Autodesk Inventor part; units mm, degrees
ref_plane "Work Plane1" through (0, 0, 1.6) normal (0, 0, 1) x (1, 0, 0)
ref_plane "Work Plane2" through (15, 0, 0) normal (1, 0, 0) x (0, 1, 0)
ref_plane "XZ Plane" through (0, 0, 0) normal (0, 1, 0) x (-1, 0, 0)
sketch "Sketch2" plane through (0, 0, 0) normal (0, 1, 0) x (-1, 0, 0)
  line L0 (0, 0) -> (-5, 0)
  line L1 (-5, 0) -> (-10, 1.6)
  line L2 (-10, 1.6) -> (-15, 1.6)
  dimension "d0" = 1.6
  dimension "d1" = 5
  dimension "d2" = 5
  dimension "d3" = 5
sketch "Sketch3" plane through (0, 0, 0) normal (1, 0, 0) x (0, 1, 0)
  circle A0 centre (0, 0) radius 0.9
  dimension "d4" = 1.8
sweep "Sweep1" add profiles "Sketch3" path "Sketch2"
ref_plane "Work Plane1" through (0, 0, 1.6) normal (0, 0, 1) x (1, 0, 0)
sketch "Sketch4" plane through (0, 0, 1.6) normal (0, 0, 1) x (1, 0, 0)
  line L0 (15, 0) -> (25, 0)
  line L1 (35.6066, -25.6066) -> (31.9289, -29.2843)
  line L2 (29, -36.3553) -> (29, -67.5)
  arc A0 (35.6066, -25.6066) -> (25, 0) centre (25, -15) ccw
  arc A1 (31.9289, -29.2843) -> (29, -36.3553) centre (39, -36.3553) ccw
  point P0 (0, 0)
  dimension "d7" = 15
  dimension "d8" = 15
  dimension "d9" = 10
  dimension "d10" = 10
  dimension "d11" = 45
  dimension "d13" = 14
  dimension "d14" = 67.5
ref_plane "Work Plane2" through (15, 0, 0) normal (1, 0, 0) x (0, 1, 0)
sketch "Sketch5" plane through (15, 0, 0) normal (1, 0, 0) x (0, 1, 0)
  circle A0 centre (0, 1.6) radius 0.9
  point P0 (0, 0)
  dimension "d16" = 1.6
  dimension "d17" = 1.8
sweep "Sweep2" add profiles "Sketch5" path "Sketch4"
sketch "Sketch7" plane through (29, -67.5, 1.6) normal (0, -1, 0) x (1, 0, 0)
  circle A0 centre (0, 0) radius 0.9
  circle A1 centre (0, 0) radius 1.2065
  point P0 (-29, -1.6)
  dimension "d21" = 2.413
extrude "Extrusion1" add sketch "Sketch7" against normal blind 3.048
sketch "Sketch8" plane through (29, -64.452, 1.6) normal (0, 1, 0) x (1, 0, 0)
  circle A0 centre (0, 0) radius 0.9
  circle A1 centre (0, 0) radius 1.2065
  circle A2 centre (0, 0) radius 1.7526
  point P0 (-29, 1.6)
  dimension "d24" = 3.5052
extrude "Extrusion2" add sketch "Sketch8" along normal blind 2.032 contours A1 | A2
sketch "Sketch9" plane through (29, -62.42, 1.6) normal (0, 1, 0) x (1, 0, 0)
  circle A0 centre (0, 0) radius 0.9
  circle A1 centre (0, 0) radius 1.7526
  circle A2 centre (0, 0) radius 1.905
  point P0 (-29, 1.6)
  dimension "d27" = 3.81
extrude "Extrusion3" add sketch "Sketch9" along normal blind 8.382 contours A1 | A2
sketch "Sketch10" plane through (29, -54.038, 1.6) normal (0, 1, 0) x (1, 0, 0)
  circle A0 centre (0, 0) radius 0.9
  circle A1 centre (0, 0) radius 1.905
  circle A2 centre (0, 0) radius 1.3462
  point P0 (-29, 1.6)
  dimension "d30" = 2.6924
extrude "Extrusion4" add sketch "Sketch10" along normal blind 17.78 contours A2
properties part number "coax_tx"
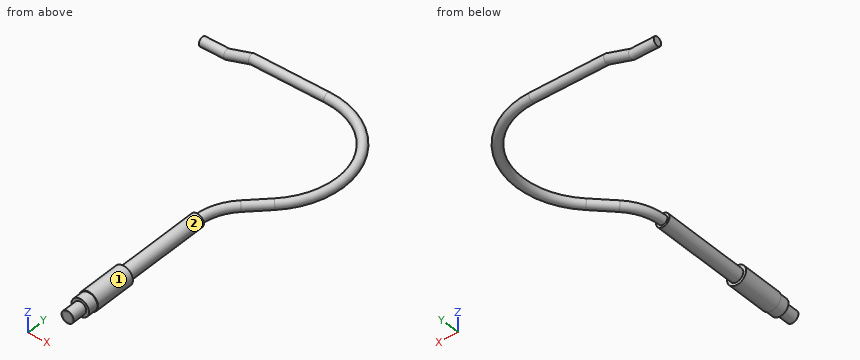
Part model, mm, in its own coordinate system. Face numbers are marked on the shaded views. Round coordinates to 2 decimals unless told otherwise and drop trailing zeros. Loops run counter-clockwise (first coordinate to the right, second up) from the corner with the lowest first, then second, coordinate; pieces in that order, holes last.
Item 1: Drop flat-ended pins along their axis: P1, Ø1.9, axis at x = 28, z = 1, coming from the +Y side; P2, Ø1.5, axis at y = -45, z = 2.5, coming from the -X side; P3, Ø10, axis at x = 31.5, y = -37.5, coming from the +Z side. Give the stop position or say it passes through.
Item 2: Cut at B-B, the plane y = -52.5. Give the cut face in (x, z).
Item 3: Mould opens along Y. For the marked faces 1 and 2 say: +Y half, -Y half, draft (parallel to the pull), parting line (faces both ways), or undercut.
Item 4: Cut at A-A, the plane x = 18.5. Give the cut face in (y, z).
Item 5: Drill centre lines: line 1 (X direction, y = -60, z = 1.85); line 2 (Y direction, x = 35.5, z = 2); line 3 (Z direction, x = 28, y = -44). Where is each one in solid material? Low to high.
A:
1. P1: stops at y = 0.74
1. P2: stops at x = 27.66
1. P3: stops at z = 2.95
2. outline: circle Ø2.69 at (29, 1.6)
3. face 1: draft
3. face 2: undercut
4. outline: circle Ø1.8 at (0, 1.6)
5. line 1: x = 27.11 to 30.89
5. line 2: y = -26.85 to -24.55, -5.45 to -3.19
5. line 3: z = 0.7 to 2.5
